```python
from build123d import *

# Parameters (mm, degrees)
BOSS_EXTRUDE1_DEPTH = 220
SKETCH2_R           = 3.75
CUT_EXTRUDE1_DEPTH  = 5.3
SKETCH3_R           = 2.25
CUT_EXTRUDE2_DEPTH  = 221.245522088
CHAMFER1_SIZE       = 0.5


# Read off the part's stored shape, not the designer's step: LPattern1
with BuildPart() as part:
    # Sketch1 → Boss-Extrude1 (new body)
    with BuildSketch(Plane.XY):
        with BuildLine():
            Line((-5.587867966, 4.655032034), (-7.353553391, 2.889346609))
            ThreePointArc((-7.353553391, 2.889346609), (-7.461939766, 2.727134935), (-7.5, 2.535793219))
            Line((-7.5, 2.535793219), (-7.5, 0.7))
            Line((-7.5, 0.7), (-6.8, 0))
            Line((-6.8, 0), (6.8, 0))
            Line((6.8, 0), (7.5, 0.7))
            Line((7.5, 0.7), (7.5, 2.535793219))
            ThreePointArc((7.5, 2.535793219), (7.461939766, 2.727134935), (7.353553391, 2.889346609))
            Line((7.353553391, 2.889346609), (5.587867966, 4.655032034))
            ThreePointArc((5.587867966, 4.655032034), (5.52283614, 4.752359039), (5.5, 4.867164069))
            Line((5.5, 4.867164069), (5.5, 7.007735931))
            ThreePointArc((5.5, 7.007735931), (5.52283614, 7.122540961), (5.587867966, 7.219867966))
            Line((5.587867966, 7.219867966), (6.022194074, 7.654194074))
            ThreePointArc((6.022194074, 7.654194074), (6.08029105, 7.736033047), (6.108143767, 7.832454529))
            ThreePointArc((6.108143767, 7.832454529), (6.479087517, 8.641867539), (7.257052023, 9.074903237))
            ThreePointArc((7.257052023, 9.074903237), (7.431425589, 9.178529998), (7.5, 9.369428391))
            Line((7.5, 9.369428391), (7.5, 10.830571609))
            ThreePointArc((7.5, 10.830571609), (7.431425589, 11.021470002), (7.257052023, 11.125096763))
            ThreePointArc((7.257052023, 11.125096763), (6.568589176, 11.46951378), (6.158449701, 12.120965838))
            ThreePointArc((6.158449701, 12.120965838), (6.128637664, 12.188930096), (6.0830537, 12.2474963))
            Line((6.0830537, 12.2474963), (5.918417966, 12.412132034))
            ThreePointArc((5.918417966, 12.412132034), (5.821090961, 12.47716386), (5.706285931, 12.5))
            Line((5.706285931, 12.5), (-5.706285931, 12.5))
            ThreePointArc((-5.706285931, 12.5), (-5.821090961, 12.47716386), (-5.918417966, 12.412132034))
            Line((-5.918417966, 12.412132034), (-6.0830537, 12.2474963))
            ThreePointArc((-6.0830537, 12.2474963), (-6.128637664, 12.188930096), (-6.158449701, 12.120965838))
            ThreePointArc((-6.158449701, 12.120965838), (-6.568589176, 11.46951378), (-7.257052023, 11.125096763))
            ThreePointArc((-7.257052023, 11.125096763), (-7.431425589, 11.021470002), (-7.5, 10.830571609))
            Line((-7.5, 10.830571609), (-7.5, 9.369428391))
            ThreePointArc((-7.5, 9.369428391), (-7.431425589, 9.178529998), (-7.257052023, 9.074903237))
            ThreePointArc((-7.257052023, 9.074903237), (-6.479087517, 8.641867539), (-6.108143767, 7.832454529))
            ThreePointArc((-6.108143767, 7.832454529), (-6.08029105, 7.736033047), (-6.022194074, 7.654194074))
            Line((-6.022194074, 7.654194074), (-5.587867966, 7.219867966))
            ThreePointArc((-5.587867966, 7.219867966), (-5.52283614, 7.122540961), (-5.5, 7.007735931))
            Line((-5.5, 7.007735931), (-5.5, 4.867164069))
            ThreePointArc((-5.5, 4.867164069), (-5.52283614, 4.752359039), (-5.587867966, 4.655032034))
        make_face()
    extrude(amount=BOSS_EXTRUDE1_DEPTH)

    # Sketch2 → Cut-Extrude1 (cut)
    with BuildSketch(Plane(origin=(0, 12.5, 0), x_dir=(1, 0, 0), z_dir=(0, 1, 0))):
        with Locations(Location((0, -10, 0), (0, 0, 270))):
            Circle(SKETCH2_R)
    extrude(amount=-CUT_EXTRUDE1_DEPTH, mode=Mode.SUBTRACT)

    # Sketch3 → Cut-Extrude2 (cut, through all)
    with BuildSketch(Plane(origin=(0, 7.2, 0), x_dir=(1, 0, 0), z_dir=(0, 1, 0))):
        with Locations(Location((0, -10, 0), (0, 0, 270))):
            Circle(SKETCH3_R)
    extrude(amount=-CUT_EXTRUDE2_DEPTH, mode=Mode.SUBTRACT)

    # Chamfer1
    chamfer1_edges = [part.edges().sort_by_distance(p)[0] for p in [
        (0, 12.5, 6.25),
        (0, 0, 7.75),
    ]]
    chamfer(chamfer1_edges, length=CHAMFER1_SIZE)

    # LPattern1 outline → LPattern1 (revolve, cut)
    with BuildSketch(Plane.XY.offset(190)):
        Polygon((0, 0), (2.75, 0), (2.25, 0.5), (2.25, 7.2), (3.75, 7.2), (3.75, 12), (4.25, 12.5), (0, 12.5), align=None)
    revolve(axis=Axis((0, 0, 190), (0, 1, 0)), mode=Mode.SUBTRACT)

    # LPattern1 2 outline → LPattern1 2 (revolve, cut)
    with BuildSketch(Plane.XY.offset(130)):
        Polygon((0, 12.5), (0, 0), (2.75, 0), (2.25, 0.5), (2.25, 7.2), (3.75, 7.2), (3.75, 12), (4.25, 12.5), align=None)
    revolve(axis=Axis((0, 0, 130), (0, 1, 0)), mode=Mode.SUBTRACT)

    # LPattern1 3 outline → LPattern1 3 (revolve, cut)
    with BuildSketch(Plane.XY.offset(70)):
        Polygon((0, 12.5), (0, 0), (2.75, 0), (2.25, 0.5), (2.25, 7.2), (3.75, 7.2), (3.75, 12), (4.25, 12.5), align=None)
    revolve(axis=Axis((0, 0, 70), (0, 1, 0)), mode=Mode.SUBTRACT)


solid = part.part
```
Here's how the part is built. I have some questions about the finished solid (model axes, mm). A direction names the side the tool comes from. Give positions to 0.01 mm unless a question says otherwise; leave off trailing zeros. Use one line per item in the form item = value.
1) I'm going to push flat-ended pins straight in: pin 1 (4 mm diameter, centred on x = -1.5, z = 190.5, fed in from +Y); pin 2 (3.5 mm diameter, centred on x = 0, z = 130, fed in from -Y); pin 3 (1.7 mm diameter, centred on y = 5.5, z = 156, fed in from +X); pin 4 (6 mm diameter, centred on x = 0.5, z = 11.5, fed in from +Y). Where does each tip first touch, or does it pass through?
Verdict:
pin_1 = 7.2
pin_2 = through
pin_3 = 5.59
pin_4 = 12.5
2) If I drill on L1, parallel to Z at x = 3, y = 9.5; L2, parallel to X at y = 4.75, z = 130; L3, parallel to X at y = 2.25, z = 130, over which ranges is the centre line in solid material (lowest first)? Write a range as [from, to].
Verdict:
L1 = [0, 7.75], [12.25, 67.75], [72.25, 127.75], [132.25, 187.75], [192.25, 220]
L2 = [-5.52, -2.25], [2.25, 5.52]
L3 = [-7.5, -2.25], [2.25, 7.5]
3) On a 3-axis mill with a long thin cutter (end or side, diameter ignored), from which of +Z, -Z, +X, -X, +Y, -Y can I reach the whole of each face in a straight line? I mean faces 1 (the face through (-0.488, 3.897, 72.196)), 2 (the face through (-0.488, 9.634, 66.282)). Say none if no direction works.
Verdict:
face_1 = +Y, -Y
face_2 = +Y
4) We'd pull the mould along X, two halves only. Please class faces 3 (the face through (-0.81, 9.63, 133.66)), 4 (the face through (0, 12.5, 108)): +X half, -X half, draft (parallel to the pull), parting line (faces both ways), or undercut.
Verdict:
face_3 = undercut
face_4 = draft
5) Suppose I cut it at A-A (x = 0). Give the number of separate pieces and of enclosed holes in the cut face, and give its area (3 significant figures).
Verdict:
separate_pieces = 5
enclosed_holes = 0
area = 2,460 mm2
